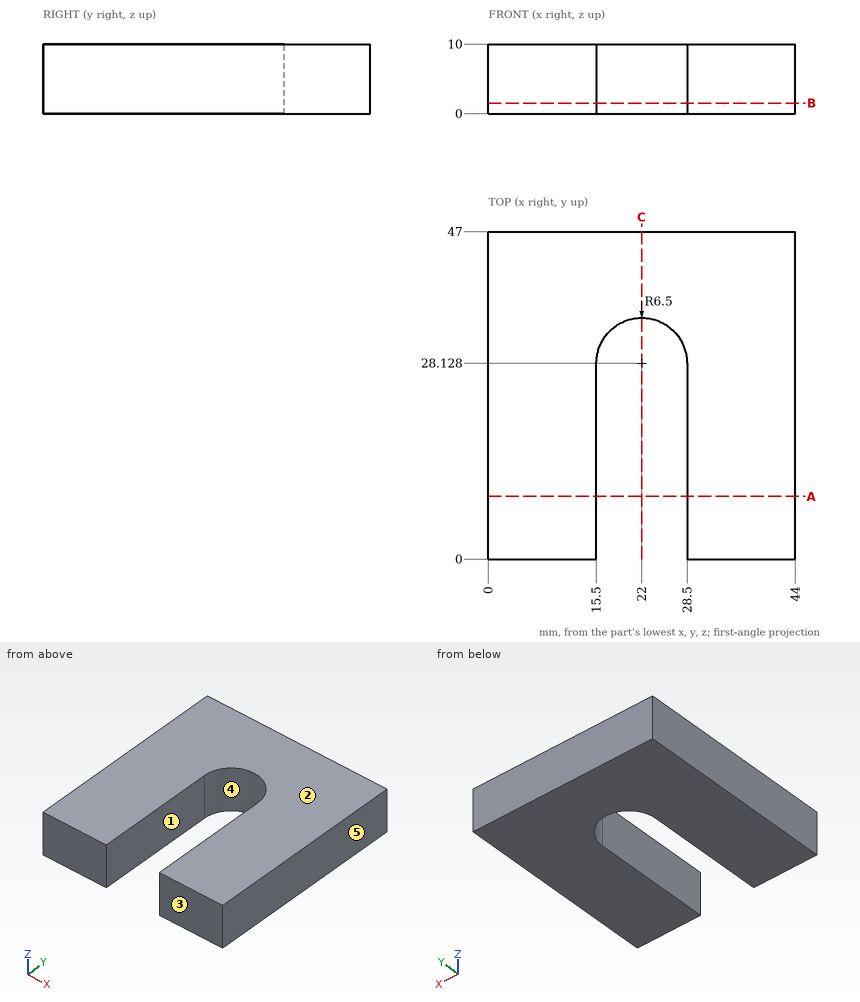
Answer from the drawing. Dimensions are ordinates in mm from the lowest x, y and z of the part. A direction names the side the tool comes from. Coordinates: 2 decimals unless noted, no trailing zeros. Write each loop counter-clockwise with the first axis right and the second up, starting at its lowest first coordinate (ties: lowest second). Pieces come first, ordered by that corner, then holes. Notation, with made-up numbers: (70.25, 79) - (87.25, 79) arc R22 ccw to (87.25, 111) - close; hole circle Ø6 at (79, 36.5). An arc over 180 degrees is marked (long way). Return JSON: item names as keys, results as strings.
1. The part is cut by section C-C on x = 22. Determine the outline of the cut face in (y, z).
Final values:
{"outline": "(34.63, 0) - (47, 0) - (47, 10) - (34.63, 10) - close"}
2. For a pull along X with two mould halves and no side action, classify the marked faces 3, 4 and 5 as +X half, -X half, draft (parallel to the pull), parting line (faces both ways), or undercut.
Final values:
{"face 3": "draft", "face 4": "undercut", "face 5": "+X half"}
3. The part is cut by section B-B on z = 1.5. Determine the outline of the cut face in (x, y), then the cut area to 3 significant figures.
Final values:
{"outline": "(0, 0) - (15.5, 0) - (15.5, 28.13) arc R6.5 cw to (28.5, 28.13) - (28.5, 0) - (44, 0) - (44, 47) - (0, 47) - close", "area": "1,640 mm^2"}
4. The part is cut by section A-A on y = 9. Determine the outline of the cut face in (x, z).
Final values:
{"outline": "(0, 0) - (15.5, 0) - (15.5, 10) - (0, 10) - close; (28.5, 0) - (44, 0) - (44, 10) - (28.5, 10) - close"}
5. This flat-tipped pin is pushed along its axis until it touches: pin 1 Ø4 at (x, z) = (20.5, 3) entering from -Y (1 decimal). Where does it stop, or does it pass through?
Final values:
{"pin 1": "y = 33.6"}
6. Which of the six approach directions +Z, -Z, +X, -X, +Y, -Y give full straight-line access (tool end or side, diameter ignored) to the marked faces 1 and 2?
Final values:
{"face 1": "+Z, -Z, -Y", "face 2": "+Z, +X, -X, +Y, -Y"}
7. Consider line 1 along X through (y, z) = (11, 6.5); line 2 along X through (y, z) = (33, 5.25); line 3 along Y through (x, z) = (19.5, 5). Determine where each line is inside the solid, lowest interval first.
Final values:
{"line 1": "0 to 15.5, 28.5 to 44", "line 2": "0 to 17.7, 26.3 to 44", "line 3": "34.13 to 47"}
